Input: part model. Units: mm. Frame: model coordinates. Face numbers are marked on the shaded views. A direction names the side the tool comes from. Coordinates: 2 decimals unless noted, no trailing zeros. Write each loop counter-clockwise with the first axis right and the second up, starting at its lowest first coordinate (ties: lowest second). Pieces come first, ordered by that corner, then holes. Notation, with made-up numbers: (30.5, -37) -> (89.5, -37) arc R14 cw to (89.5, -19) -> close; hole circle Ø9 at (65, -29). An arc over 180 degrees is marked (long way). Use one line per item in the form item = value. Start each with the question number.
(1) Set-up query: the marked faces 4 and 5. Return all of +Z, -Z, +X, -X, +Y, -Y with unobstructed straight access to the full face (end or side cutting, diameter ignored); none if empty.
(2) Pull-direction query (X, two-part tool) for the marked faces 1, 2 and 3; classes: released by +X, released by -X, zero draft, split by the parting line, or undercut.
(3) Cut plane D-D on y = -7.7. Return the cut outline in (x, z).
(4) First-contact query: pin 1 (5 mm diameter, centred on x = 0, y = -12, fed in from +Z); pin 2 (1 mm diameter, centred on x = 5.5, z = 0.5, fed in from -Y). Flat tips, straight axial feed; report the tip coordinate or a pass-through.
(5) Ray query, line 1 along Y through (x, z) = (-0.5, 0.6); line 2 along X through (y, z) = (1.5, 0.2); line 3 along Y through (x, z) = (0.5, 1.8). Return the intervals inside material, ascending.
(6) Cut plane C-C on x = 6. Return the cut outline in (y, z).
(7) Cut plane A-A on x = 0. Return the cut outline in (y, z), plus the area to 3 significant figures.
(8) Cut plane B-B on y = -2.5. Return the cut outline in (x, z), plus the area to 3 significant figures.
```python
from build123d import *

# Parameters (mm, degrees)
SKETCH_1_W          = 24
SKETCH_1_H          = 33.932299882
SKETCH_1_R          = 1.5
SKETCH_1_R_2        = 6.44
SKETCH_1_R_3        = 3
EXTRUDE_1_DEPTH     = 2
CUT_EXTRUDE_START   = 2
SKETCH_1_3_R        = 3
SKETCH_1_3_R_2      = 1.5
CUT_EXTRUDE_1_DEPTH = 1
SKETCH_2_W          = 24
SKETCH_2_H          = 33.932299882
CUT_EXTRUDE_3_DEPTH = 3


with BuildPart() as part:
    # 草图1 → 凸台-拉伸1 (new body)
    with BuildSketch(Plane.XY):
        with Locations((0, -4.966149941)):
            Rectangle(SKETCH_1_W, SKETCH_1_H)
        with Locations((-8.75, -7.7)):
            Circle(SKETCH_1_R, mode=Mode.SUBTRACT)
        Circle(SKETCH_1_R_2, mode=Mode.SUBTRACT)
        with Locations((0, -12)):
            Circle(SKETCH_1_R_3, mode=Mode.SUBTRACT)
        with Locations((8.75, -7.7)):
            Circle(SKETCH_1_R, mode=Mode.SUBTRACT)
        with Locations((0, -12)):
            Circle(SKETCH_1_R_3)
        with Locations((0, -12)):
            Circle(SKETCH_1_R, mode=Mode.SUBTRACT)
    extrude(amount=EXTRUDE_1_DEPTH)

    # 草图1<3> → 切除-拉伸1 (cut)
    with BuildSketch(Plane.XY.offset(CUT_EXTRUDE_START)):
        with Locations((0, -12)):
            Circle(SKETCH_1_3_R)
        with Locations((0, -12)):
            Circle(SKETCH_1_3_R_2, mode=Mode.SUBTRACT)
    extrude(amount=-CUT_EXTRUDE_1_DEPTH, mode=Mode.SUBTRACT)

    # 草图2 → 切除-拉伸3 (cut, through all)
    with BuildSketch(Plane.XY.offset(2)):
        with Locations((0, -4.966149941)):
            Rectangle(SKETCH_2_W, SKETCH_2_H)
        with BuildLine():
            ThreePointArc((-10.616967552, -4.419275959), (0, -20.338551918), (10.616967552, -4.419275959))
            ThreePointArc((10.616967552, -4.419275959), (0, 11.5), (-10.616967552, -4.419275959))
        make_face(mode=Mode.SUBTRACT)
    extrude(amount=-CUT_EXTRUDE_3_DEPTH, mode=Mode.SUBTRACT)


solid = part.part
```
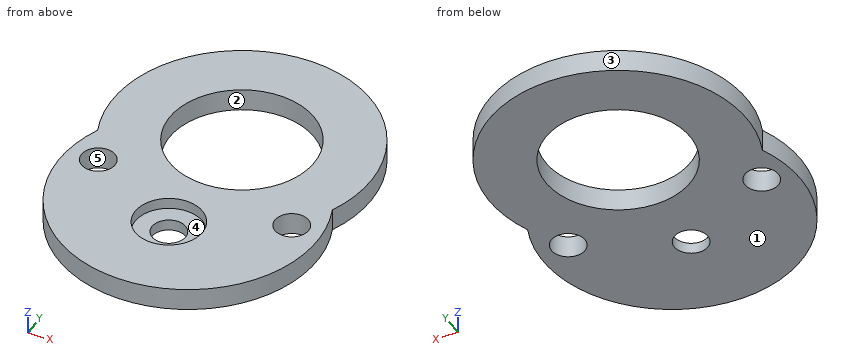
Values:
q1.face_4 = +Z
q1.face_5 = +Z, -Z
q2.face_1 = zero draft
q2.face_2 = undercut
q2.face_3 = split by the parting line
q3.outline = (-11.44, 0) -> (-10.25, 0) -> (-10.25, 2) -> (-11.44, 2) -> close; (-7.25, 0) -> (7.25, 0) -> (7.25, 2) -> (-7.25, 2) -> close; (10.25, 0) -> (11.44, 0) -> (11.44, 2) -> (10.25, 2) -> close
q4.pin_1 = 1
q4.pin_2 = -19.19
q5.line_1 = -20.33 to -13.41, -10.59 to -6.42, 6.42 to 11.49
q5.line_2 = -11.4 to -6.26, 6.26 to 11.4
q5.line_3 = -20.33 to -14.96, -9.04 to -6.42, 6.42 to 11.49
q6.outline = (-18.65, 0) -> (-2.34, 0) -> (-2.34, 2) -> (-18.65, 2) -> close; (2.34, 0) -> (9.81, 0) -> (9.81, 2) -> (2.34, 2) -> close
q7.outline = (-20.34, 0) -> (-13.5, 0) -> (-13.5, 1) -> (-15, 1) -> (-15, 2) -> (-20.34, 2) -> close; (-10.5, 0) -> (-6.44, 0) -> (-6.44, 2) -> (-9, 2) -> (-9, 1) -> (-10.5, 1) -> close; (6.44, 0) -> (11.5, 0) -> (11.5, 2) -> (6.44, 2) -> close
q7.area = 28.9 mm2
q8.outline = (-11.22, 0) -> (-5.93, 0) -> (-5.93, 2) -> (-11.22, 2) -> close; (5.93, 0) -> (11.22, 0) -> (11.22, 2) -> (5.93, 2) -> close
q8.area = 21.2 mm2
